```python
from build123d import *

# Parameters (mm, degrees)
BOSS_EXTRUDE1_DEPTH = 3
SKETCH4_R           = 1.55
SKETCH4_W           = 9
SKETCH4_H           = 5.2
SKETCH4_W_2         = 14
CUT_EXTRUDE1_DEPTH  = 3


with BuildPart() as part:
    # Sketch1 → Boss-Extrude1 (new body)
    with BuildSketch(Plane(origin=(0, 0, 0), x_dir=(-1, 0, 0), z_dir=(0, 0, 1))):
        Polygon((-3.476318152, -7.837615564), (-3.476318152, -4.837615564), (6.523681848, -4.837615564), (6.523681848, -7.837615564), (26.523681848, -7.837615564), (26.523681848, -14.837615564), (29.523681848, -14.837615564), (29.523681848, -24.837615564), (26.523681848, -24.837615564), (26.523681848, -32.337615564), (6.523681848, -32.337615564), (6.523681848, -35.337615564), (-3.476318152, -35.337615564), (-3.476318152, -32.337615564), (-23.476318152, -32.337615564), (-23.476318152, -24.837615564), (-26.476318152, -24.837615564), (-26.476318152, -14.837615564), (-23.476318152, -14.837615564), (-23.476318152, -7.837615564), align=None)
    extrude(amount=BOSS_EXTRUDE1_DEPTH)

    # Sketch4 → Cut-Extrude1 (cut)
    with BuildSketch(Plane.XY.offset(3)):
        with Locations((13.476318152, 15.437615564)):
            Circle(SKETCH4_R)
        with Locations(Location((-16.523681848, 15.437615564, 0), (0, 0, 180))):
            Circle(SKETCH4_R)
        with Locations((-0.023681848, 12.937615564)):
            Rectangle(SKETCH4_W, SKETCH4_H)
        with Locations((11.976318152, 24.237615564)):
            Rectangle(SKETCH4_W, SKETCH4_H)
        with Locations((-14.523681848, 24.237615564)):
            Rectangle(SKETCH4_W_2, SKETCH4_H)
    extrude(amount=-CUT_EXTRUDE1_DEPTH, mode=Mode.SUBTRACT)


solid = part.part
```
Model file for the job. Use its own axes, mm. A direction names the side the tool comes from. Coordinates: 2 decimals unless noted, no trailing zeros. Order: outer loops, then holes, each group sorted by start corner. A loop starts at its lowest first (then second) coordinate and runs counter-clockwise, first axis right, second up. Notation, with made-up numbers: (80.5, 67) - (104.5, 67) arc R24 ccw to (104.5, 99) - close; hole circle Ø8 at (36, 48). An arc over 180 degrees is marked (long way). Return JSON: item names as keys, results as strings. Group by question number.
1) Saw through at A-A, the plane y = 12. Write the cut outline in (x, z).
2) Saw through at B-B, the plane x = 0.5. Write the cut outline in (y, z).
3) Tool access for faces 1 (the flat face through (3.476, 6, 1)), 2 (the flat face through (25, 24.838, 1)), 3 (the flat face through (-28, 14.838, 1)), 4 (the flat face through (-4.524, 13, 2)): list every direction of +Z, -Z, +X, -X, +Y, -Y with a clear straight run to the whole face (end or side of a thin tool).
4) Probe line 1 (X direction, y = 15.5, z = 1.9); line 2 (Y direction, x = -19.5, z = 0.15); line 3 (X direction, y = 10.5, z = 1). List the from-to ranges inside material, lowest first. Write a range as from..to.
5) Saw through at D-D, the plane y = 30.5. Write the cut outline in (x, z), plus the area to 3 significant figures.
6) Flat gauge pins, fed straight in: P1, Ø3, axis at x = 5, y = 16, coming from the -Z side; P2, Ø0.9, axis at x = -28.5, z = 1.5, coming from the +Y side; P3, Ø0.9, axis at x = -28, z = 1.5, coming from the -Y side; P4, Ø0.9, axis at x = -14, z = 1.5, coming from the -Y side. Where does each tip first touch, or does it go through?
7) Mould opens along Y. For faces 5 (the flat face through (-26.524, 29, 1)), 6 (the flat face through (13, 32.338, 1)), 7 (the flat face through (-16, 7.838, 1)), 8 (the flat face through (-7.524, 24, 2)) say: released by +Y, released by -Y, zero draft, split by the parting line, or undercut.
8) Saw through at C-C, the plane z = 1.2. Count the separate pieces of the cut face and the enclosed holes in it, plus the area to 3 significant figures.
Values found:
{
 "1": {"outline": "(-26.52, 0) - (-4.52, 0) - (-4.52, 3) - (-26.52, 3) - close; (4.48, 0) - (23.48, 0) - (23.48, 3) - (4.48, 3) - close"},
 "2": {"outline": "(4.84, 0) - (10.34, 0) - (10.34, 3) - (4.84, 3) - close; (15.54, 0) - (35.34, 0) - (35.34, 3) - (15.54, 3) - close"},
 "3": {"face 1": "+Z, -Z, +X, -Y", "face 2": "+Z, -Z, +X, +Y", "face 3": "+Z, -Z, -X, -Y", "face 4": "+Z, -Z"},
 "4": {"line 1": "x = -29.52..-18.07, -14.97..-4.52, 4.48..11.93, 15.03..26.48", "line 2": "y = 7.84..21.64, 26.84..32.34", "line 3": "x = -26.52..-4.52, 4.48..23.48"},
 "5": {"outline": "(-26.52, 0) - (23.48, 0) - (23.48, 3) - (-26.52, 3) - close", "area": "150 mm²"},
 "6": {"P1": "stops at z = 0", "P2": "stops at y = 24.84", "P3": "stops at y = 14.84", "P4": "stops at y = 7.84"},
 "7": {"face 5": "zero draft", "face 6": "released by +Y", "face 7": "released by -Y", "face 8": "undercut"},
 "8": {"separate pieces": "1", "enclosed holes": "5", "area": "1,160 mm²"}
}
